Input: part model. Units: mm. Frame: model coordinates. A direction names the side the tool comes from. Coordinates: 2 decimals unless noted, no trailing zeros. Loops run counter-clockwise (first coordinate to the right, second up) from the corner with the lowest first, then second, coordinate; pieces in that order, holes last.
Item 1: Ray query, line 1 along Z through (x, y) = (-0.25, -10.75); line 2 along Y through (x, z) = (0, 10.5); line 3 along Z through (x, y) = (7.75, 12.25). Return the intervals inside material, ascending.
Item 2: Section A-A on z = 4. Return loops of the section in (x, y), and give its area (3 significant figures).
Item 3: Contact query for flat-ended pins moving along their axis: P1, Ø6, axis at x = 7, y = 6.5, coming from the -Z side; P2, Ø4, axis at y = -0.5, z = 18, coming from the +X side; P3, Ø4, axis at y = 9.5, z = 16.5, coming from the +X side; P4, Ø6, axis at x = -8.5, z = 15.5, coming from the -Y side. Output: stop coordinate, or through.
Item 4: Reachability of faces 1 (the flat face through (2, -8, 1)), 2 (the cylindrical face through (-14.985, 0.66, 23.732)), 3 (the flat face through (-3, 10, 22.5)) from +Z, -Z, +X, -X, +Y, -Y: full face, straight path, thin tool, end or side. Return the list, or none.
Item 5: Pull-direction query (Y, two-part tool) for faces 4 (the flat face through (2, -8, 24)), 5 (the cylindrical face through (-10, 0, 12)), 6 (the flat face through (-0.1, 13.4, 25)); classes: released by +Y, released by -Y, zero draft, split by the parting line, or undercut.
```python
from build123d import *

# Parameters (mm, degrees)
CROQUIS1_R                 = 15
CROQUIS1_R_2               = 5
SALIENTE_EXTRUIR1_DEPTH    = 25
CROQUIS3_W                 = 20
CROQUIS3_H                 = 10
CROQUIS4_R                 = 13
CROQUIS4_R_2               = 7
CORTAR_EXTRUIR1_DEPTH      = 1
CHAFL_N1_SIZE              = 1
CHAFL_N1_OF_SIMETR_A2_SIZE = 1


with BuildPart() as part:
    # Croquis1 → Saliente-Extruir1 (new body)
    with BuildSketch(Plane.XY):
        Circle(CROQUIS1_R)
        Circle(CROQUIS1_R_2, mode=Mode.SUBTRACT)
    extrude(amount=SALIENTE_EXTRUIR1_DEPTH)

    # Croquis3 → Cortar-Revolución1 (revolve, cut)
    with BuildSketch(Plane(origin=(0, 0, 0), x_dir=(0, 0, -1), z_dir=(1, 0, 0)), mode=Mode.PRIVATE) as cortar_revoluci_n1_sk:
        with Locations((-12.5, 15)):
            Rectangle(CROQUIS3_W, CROQUIS3_H)
    revolve(cortar_revoluci_n1_sk.sketch.rotate(Axis((0, 0, 25), (0, 0, -1)), 90), axis=Axis((0, 0, 25), (0, 0, -1)), mode=Mode.SUBTRACT)

    # Croquis4 → Cortar-Extruir1 (cut)
    with BuildSketch(Plane.XY.offset(25)):
        Circle(CROQUIS4_R)
        Circle(CROQUIS4_R_2, mode=Mode.SUBTRACT)
    cortar_extruir1 = extrude(amount=-CORTAR_EXTRUIR1_DEPTH, mode=Mode.SUBTRACT)

    # Chaflán1
    chafl_n1_edges = [part.edges().sort_by_distance(p)[0] for p in [
        (-13, 0, 24),
        (-7, 0, 24),
    ]]
    chamfer(chafl_n1_edges, length=CHAFL_N1_SIZE - 0.0001)  # a hair under: the kernel refuses the full size

    # Simetría2: Cortar-Extruir1 across plane
    add(cortar_extruir1.mirror(Plane.XY.offset(12.5)), mode=Mode.SUBTRACT)

    # Chaflán1 of Simetría2
    chafl_n1_of_simetr_a2_edges = [part.edges().sort_by_distance(p)[0] for p in [
        (-13, 0, 1),
        (-7, 0, 1),
    ]]
    chamfer(chafl_n1_of_simetr_a2_edges, length=CHAFL_N1_OF_SIMETR_A2_SIZE - 0.0001)  # a hair under: the kernel refuses the full size


solid = part.part
```
Results found:
1. line 1: z = 1 to 2.5, 22.5 to 24
1. line 2: y = -10 to -5, 5 to 10
1. line 3: z = 0 to 2.5, 22.5 to 25
2. outline: circle Ø20 at (0, 0); hole circle Ø10 at (0, 0)
2. area: 236 mm2
3. P1: stops at z = 0
3. P2: stops at x = 10
3. P3: stops at x = 6.61
3. P4: stops at y = -8.35
4. face 1: -Z
4. face 2: +Z, -Z
4. face 3: none
5. face 4: undercut
5. face 5: split by the parting line
5. face 6: zero draft
